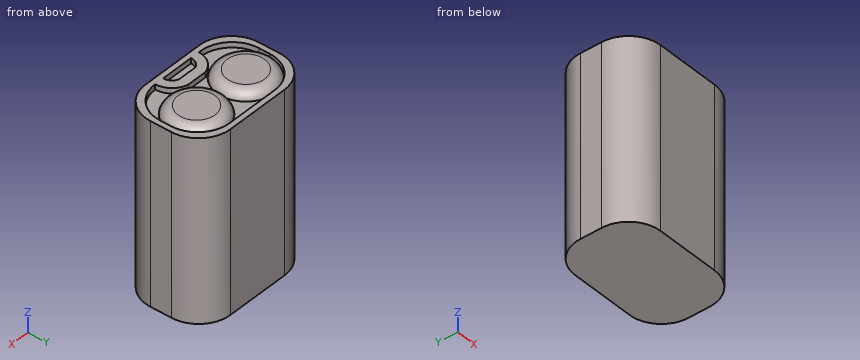
from build123d import *

# Parameters (mm, degrees)
SKETCH1_W           = 30.48
SKETCH1_H           = 43.18
BOSS_EXTRUDE1_DEPTH = 20.32
FILLET1_R           = 7.62
CUT_EXTRUDE2_DEPTH  = 1.27
SKETCH3_R           = 6.979927777
SKETCH3_R_2         = 6.904229814
BOSS_EXTRUDE2_DEPTH = 2.032
FILLET2_R           = 2.54


with BuildPart() as part:
    # Sketch1 → Boss-Extrude1 (new body)
    with BuildSketch(Plane(origin=(0, 0, 0), x_dir=(1, 0, 0), z_dir=(0, 1, 0))):
        Rectangle(SKETCH1_W, SKETCH1_H)
    extrude(amount=BOSS_EXTRUDE1_DEPTH)

    # Fillet1
    fillet1_edges = [part.edges().sort_by_distance(p)[0] for p in [
        (15.24, 20.32, 0),
        (-15.24, 20.32, 0),
        (15.24, 0, 0),
        (-15.24, 0, 0),
    ]]
    fillet(fillet1_edges, radius=FILLET1_R)

    # Sketch2 → Cut-Extrude2 (cut)
    with BuildSketch(Plane.XY.offset(21.59)):
        with BuildLine():
            Line((-3.729733948, 1.27), (4.173096077, 1.27))
            ThreePointArc((4.173096077, 1.27), (3.721271351, 2.723698057), (2.525007795, 3.66515285))
            Line((2.525007795, 3.66515285), (-2.15658026, 3.66515285))
            ThreePointArc((-2.15658026, 3.66515285), (-3.301276498, 2.702791829), (-3.729733948, 1.27))
        make_face()
        with BuildLine():
            ThreePointArc((2.645377511, 5.955761741), (5.350660012, 4.274727675), (6.407709564, 1.270218533))
            ThreePointArc((6.407709564, 1.270218533), (11.758518599, 3.522288517), (13.97, 8.89))
            Line((13.97, 8.89), (13.97, 11.43))
            ThreePointArc((13.97, 11.43), (11.738153673, 16.818153673), (6.35, 19.05))
            Line((6.35, 19.05), (-6.35, 19.05))
            ThreePointArc((-6.35, 19.05), (-11.738153673, 16.818153673), (-13.97, 11.43))
            Line((-13.97, 11.43), (-13.97, 8.89))
            ThreePointArc((-13.97, 8.89), (-11.738153673, 3.501846327), (-6.35, 1.27))
            Line((-6.35, 1.27), (-5.918912318, 1.27))
            ThreePointArc((-5.918912318, 1.27), (-4.861931172, 4.274642475), (-2.15658026, 5.955761741))
            Line((-2.15658026, 5.955761741), (2.645377511, 5.955761741))
        make_face()
    extrude(amount=-CUT_EXTRUDE2_DEPTH, mode=Mode.SUBTRACT)

    # Sketch3 → Boss-Extrude2 (add)
    with BuildSketch(Plane.XY.offset(20.32)):
        with Locations((-6.939175258, 11.673649258)):
            Circle(SKETCH3_R)
        with Locations((6.997365407, 11.673649258)):
            Circle(SKETCH3_R_2)
    extrude(amount=BOSS_EXTRUDE2_DEPTH)

    # Fillet2
    # the kernel refuses this fillet: 2.54 mm, written as the material it takes off along each edge
    with BuildSketch(Plane(origin=(-6.939175258, 11.673649258, 22.352), x_dir=(1, 0, 0), z_dir=(0, -1, 0))) as fillet2_piece_1:
        with BuildLine():
            CenterArc((4.491246199, -2.54), FILLET2_R, 11.536959033, 78.463040967)
            Line((4.491246199, 0), (6.979927777, 0))
            Line((6.979927777, 0), (6.979927777, -2.032))
        make_face()
    revolve(axis=Axis((-6.939175258, 11.673649258, 22.352), (0, 0, 1)), mode=Mode.SUBTRACT)
    with BuildSketch(Plane(origin=(6.997365407, 11.673649258, 22.352), x_dir=(1, 0, 0), z_dir=(0, -1, 0))) as fillet2_piece_2:
        with BuildLine():
            CenterArc((4.415548235, -2.54), FILLET2_R, 11.536959033, 78.463040967)
            Line((4.415548235, 0), (6.904229814, 0))
            Line((6.904229814, 0), (6.904229814, -2.032))
        make_face()
    revolve(axis=Axis((6.997365407, 11.673649258, 22.352), (0, 0, 1)), mode=Mode.SUBTRACT)


solid = part.part
The listing builds one solid part. Answer for the finished solid, in the listing's coordinates (mm). Give positions to 0.01 mm unless a question says otherwise; leave off trailing zeros. Write each loop counter-clockwise with the first axis right and the second up, starting at its lowest first coordinate (ties: lowest second). Pieces come first, ordered by that corner, then holes. Notation, with made-up numbers: (-29.75, -21) -> (-16.75, -21) arc R38 ccw to (-16.75, 18) -> close; hole circle Ø3 at (28, 19.25). An arc over 180 degrees is marked (long way). Use a Markdown table: item, result.
(1) Section A-A, the plane z = 13 is taken. Determine the outline of the cut face in (x, y), then the cut area to 3 significant figures.
Return value:
| item | result |
|---|---|
| outline | (-15.24, 7.62) arc R7.62 ccw to (-7.62, 0) -> (7.62, 0) arc R7.62 ccw to (15.24, 7.62) -> (15.24, 12.7) arc R7.62 ccw to (7.62, 20.32) -> (-7.62, 20.32) arc R7.62 ccw to (-15.24, 12.7) -> close |
| area | 570 mm2 |
(2) Find the intervals of material crossed by probe 1 along Y at (x, z) = (-8, -5); probe 2 along Z at (x, y) = (0, 2.5); probe 3 along Z at (x, y) = (12.5, 3.5), in increasing order. Write a range as from..to.
Return value:
| item | result |
|---|---|
| probe 1 | 0.01..20.31 |
| probe 2 | -21.59..20.32 |
| probe 3 | -21.59..21.59 |
(3) Section B-B, the plane y = 2 is taken. Determine the outline of the cut face in (x, z).
Return value:
| item | result |
|---|---|
| outline | (-12.77, -21.59) -> (12.77, -21.59) -> (12.77, 21.59) -> (9.6, 21.59) -> (9.6, 20.32) -> (6.35, 20.32) -> (6.35, 21.59) -> (4.07, 21.59) -> (4.07, 20.32) -> (-3.63, 20.32) -> (-3.63, 21.59) -> (-5.86, 21.59) -> (-5.86, 20.32) -> (-9.6, 20.32) -> (-9.6, 21.59) -> (-12.77, 21.59) -> close |
(4) Flat-ended cylindrical pins translate along their axes: P1, Ø1, axis at x = 1, y = 9, coming from the +Z side; P2, Ø1, axis at x = -8, y = 7, coming from the +Z side; P3, Ø0.7, axis at x = 1, y = 2, coming from the +Z side. Find the tip coordinate at first contact, or state that the pin passes through.
Return value:
| item | result |
|---|---|
| P1 | z = 21.74 |
| P2 | z = 22.35 |
| P3 | z = 20.32 |
